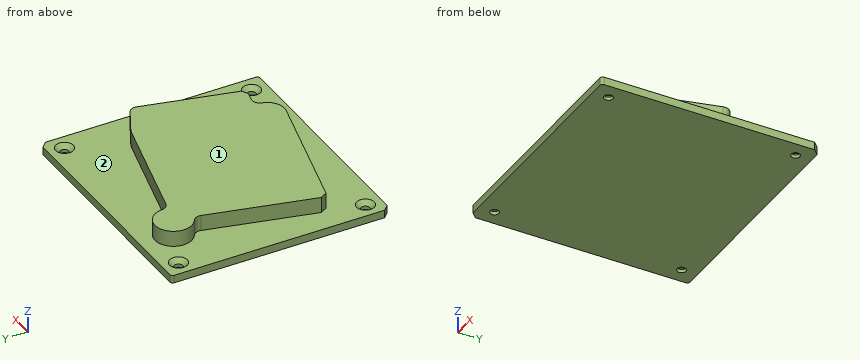
from build123d import *

# Parameters (mm, degrees)
PAD_DEPTH        = 6
HOLE_D           = 6.6
HOLE_DEPTH       = 25
HOLE_CSINK_D     = 13.44
HOLE_CSINK_ANGLE = 90
PAD001_DEPTH     = 12


with BuildPart() as part:
    # Sketch → Pad (new body)
    with BuildSketch(Plane.XY):
        with BuildLine():
            ThreePointArc((2, 166), (0.585786, 165.414214), (0, 164))
            Line((0, 164), (0, 4.242641))
            Line((0, 4.242641), (4.242641, 0))
            Line((4.242641, 0), (178, 0))
            ThreePointArc((178, 0), (179.414214, 0.585786), (180, 2))
            Line((180, 2), (180, 161.757359))
            Line((175.757359, 166), (180, 161.757359))
            Line((175.757359, 166), (2, 166))
        make_face()
    extrude(amount=PAD_DEPTH)

    # Hole
    with Locations(Plane.XY.offset(6)):
        with Locations((12, 154), (168, 154), (168, 12), (12, 12)):
            CounterSinkHole(HOLE_D / 2, HOLE_CSINK_D / 2, depth=HOLE_DEPTH, counter_sink_angle=HOLE_CSINK_ANGLE)

    # Sketch002 (on Face5 of Hole) → Pad001 (join)
    with BuildSketch(Plane.XY.offset(6)):
        with BuildLine():
            ThreePointArc((56.618237, 141.695686), (35.433188, 152.851689), (35.337576, 128.908975))
            ThreePointArc((38.028145, 122.339284), (37.758773, 126.064762), (35.337576, 128.908975))
            Line((38.028145, 122.339284), (18.026388, 42.116616))
            Line((18.026388, 42.116616), (21.116616, 36.973612))
            Line((119.851347, 12.356279), (21.116616, 36.973612))
            ThreePointArc((119.851347, 12.356279), (129.691827, 13.826949), (135.610176, 21.825139))
            ThreePointArc((142.883482, 26.195382), (138.341722, 25.516611), (135.610176, 21.825139))
            Line((149.78317, 24.475096), (142.883482, 26.195382))
            Line((149.78317, 24.475096), (154.49759, 27.307806))
            Line((171.860307, 96.945859), (154.49759, 27.307806))
            ThreePointArc((171.860307, 96.945859), (171.519804, 100.837813), (168.855356, 103.695079))
            Line((151.638919, 112.849221), (168.855356, 103.695079))
            ThreePointArc((151.638919, 112.849221), (148.639117, 114.216311), (145.495068, 115.207626))
            Line((145.495068, 115.207626), (61.155784, 136.235771))
            ThreePointArc((56.618237, 141.695686), (57.992845, 138.222619), (61.155784, 136.235771))
        make_face()
    extrude(amount=PAD001_DEPTH)


solid = part.part
Check sheet for the modelled part. Datum: model origin and axes. Units: mm. Face numbers are marked on the shaded views. A direction names the side the tool comes from. Round coordinates to 2 decimals unless told otherwise and drop trailing zeros. Order: outer loops, then holes, each group sorted by start corner. A loop starts at its lowest first (then second) coordinate and runs counter-clockwise, first axis right, second up.
Q1. Cross-section at B-B, the plane z = 10. Enter the section's corners in (x, y), plus the area to 3 significant figures.
Filled sheet:
outline: (18.03, 42.12) - (21.12, 36.97) - (119.85, 12.36) arc R13 ccw to (135.61, 21.83) arc R6 cw to (142.88, 26.2) - (149.78, 24.48) - (154.5, 27.31) - (171.86, 96.95) arc R6 ccw to (168.86, 103.7) - (151.64, 112.85) arc R27 ccw to (145.5, 115.21) - (61.16, 136.24) arc R6 cw to (56.62, 141.7) arc R14 ccw (long way) to (35.34, 128.91) arc R6 cw to (38.03, 122.34) - close
area: 14,400 mm2
Q2. Depth check by flat-ended pin: P1, Ø12, axis at x = 129, y = 70, coming from the -Z side; P2, Ø1.5, axis at x = 115.5, z = 8.5, coming from the +Y side; P3, Ø1.5, axis at y = 57.5, z = 11.5, coming from the -X side; P4, Ø4, axis at y = 107.5, z = 10, coming from the -X side. Enter the tip coordinate at first touch or a pass-through.
Filled sheet:
P1: stops at z = 0
P2: stops at y = 122.87
P3: stops at x = 21.67
P4: stops at x = 33.83
Q3. Scan lines: L1, parallel to Y at x = 12, z = 1.2; L2, parallel to X at y = 154, z = 1.65; L3, parallel to Z at x = 169, y = 135.5. Record each from-to range of solid material in increasing order.
Filled sheet:
L1: y = 0 to 8.7, 15.3 to 150.7, 157.3 to 166
L2: x = 0 to 8.7, 15.3 to 164.7, 171.3 to 180
L3: z = 0 to 6
Q4. Cross-section at D-D, the plane x = 78. Enter the section's corners in (y, z).
Filled sheet:
outline: (0, 0) - (166, 0) - (166, 6) - (132.04, 6) - (132.04, 18) - (22.79, 18) - (22.79, 6) - (0, 6) - close
Q5. Set-up check for the marked faces 1 and 2: record each of +Z, -Z, +X, -X, +Y, -Y from which the full face is reachable in a straight line by a thin tool's end or side.
Filled sheet:
face 1: +Z, +X, -X, +Y, -Y
face 2: +Z
Q6. Cross-section at C-C, the plane y = 133. Enter the section's corners in (x, z).
Filled sheet:
outline: (0, 0) - (180, 0) - (180, 6) - (74.13, 6) - (74.13, 18) - (31.05, 18) - (31.05, 6) - (0, 6) - close
Q7. Cross-section at A-A, the plane x = 12. Enter the section's corners in (y, z), plus the area to 3 significant figures.
Filled sheet:
outline: (0, 0) - (8.7, 0) - (8.7, 2.58) - (5.28, 6) - (0, 6) - close; (15.3, 0) - (150.7, 0) - (150.7, 2.58) - (147.28, 6) - (18.72, 6) - (15.3, 2.58) - close; (157.3, 0) - (166, 0) - (166, 6) - (160.72, 6) - (157.3, 2.58) - close
area: 893 mm2
